The model under review builds one solid part; all positions refer to its coordinate system, in mm. Face numbers are marked on the shaded views. A direction names the side the tool comes from. Give positions to 0.01 mm unless a question says otherwise; leave off trailing zeros. Put each result on its own line as item: value. Start each with the question number.
from build123d import *


with BuildPart() as f2:
    # F2: sweep along a path in F1
    with BuildLine(Plane.XY) as f2_path:
        ThreePointArc((945.2663377975, 1277.1216029536), (512.5198472769, 1160.6314502419), (146.3091123304, 902.3115355107))
        Line((146.3091123304, 902.3115355107), (78.7500915689, 828.5838018297))
        ThreePointArc((78.7500915689, 828.5838018297), (-146.6694692914, 441.2525452569), (-225, 0))
    # F0 (on Front) → F2 (sweep)
    with BuildSketch(Plane.XZ):
        Polygon((-225, 0), (0, 0), (0, 5), (-220, 5), (-220, 430), (-225, 430), align=None)
    sweep(path=f2_path.line, transition=Transition.RIGHT)


solid = f2.part
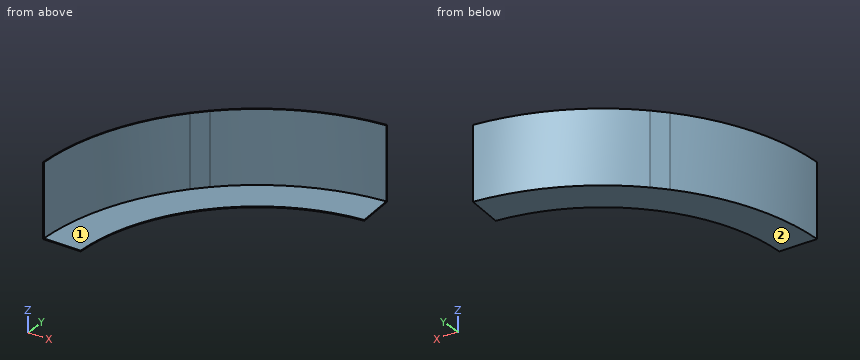
(1) For the marked faces 1 and 2, list the 3-axis set-ups (+Z, -Z, +X, -X, +Y, -Y) from which the entire face can be reached by the end or side of a thin tool; tool diameter is ignored.
(2) Insertion check: pin 1 (2 mm diameter, centred on y = 347.5, z = 364, fed in from -X); pin 2 (12 mm diameter, centred on x = 155, z = 220.5, fed in from -Y); pin 3 (5 mm diameter, centred on y = 307, z = 55.5, fed in from -X). Each pin has a flat end and moves straight along its axis. Give the tip position at first contact, or say it passes through.
(3) To check wall thickness, follow L1, parallel to Z at x = 245.5, y = 923; L2, parallel to Y at x = 120.5, z = 62; L3, parallel to Y at x = 905, z = 339.5. State the ranges of each line that lie inside material, in increasing order. Write a range as [from, to].
Check sheet entries:
1. face 1: +Z, +X, -Y
1. face 2: -Z, +X, -X, +Y, -Y
2. pin 1: stops at x = -177.29
2. pin 2: stops at y = 897.85
2. pin 3: stops at x = -188.31
3. L1: z = [0, 5]
3. L2: y = [866.74, 874.15]
3. L3: y = [1267.92, 1272.96]
